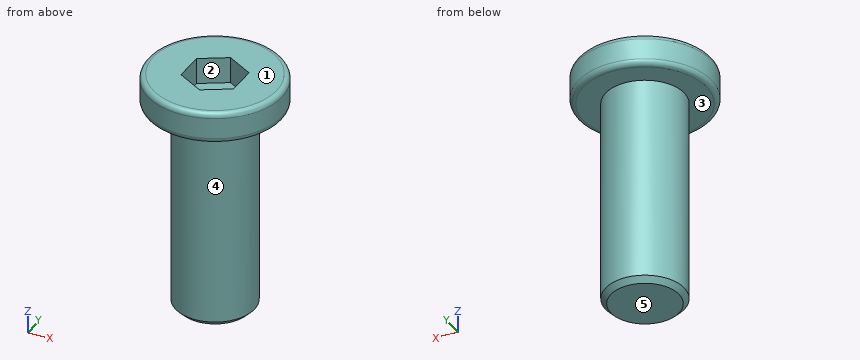
Autodesk Inventor part; units mm, degrees
ref_plane "YZ Plane" through (0, 0, 0) normal (1, 0, 0) x (0, 1, 0)
ref_plane "XZ Plane" through (0, 0, 0) normal (0, 1, 0) x (-1, 0, 0)
ref_plane "XY Plane" through (0, 0, 0) normal (0, 0, 1) x (1, 0, 0)
sketch "スケッチ1" plane through (0, 0, 0) normal (0, 0, 1) x (1, 0, 0)
  circle A0 centre (0, 0) radius 2.55
  dimension "d0" = 5.1
extrude "押し出し1" add sketch "スケッチ1" along normal blind 1.2
sketch "スケッチ2" plane through (0, 0, 0) normal (0, 0, -1) x (-1, 0, 0)
  circle A0 centre (0, 0) radius 2.55
  circle A1 centre (0, 0) radius 1.5
  dimension "d3" = 3
extrude "押し出し2" add sketch "スケッチ2" along normal blind 8 contours A1
thread "ねじ1"
sketch "スケッチ3" plane through (0, 0, 1.2) normal (0, 0, 1) x (1, 0, 0)
  circle A0 centre (0, 0) radius 2.55
  line L0 (0, 1.1547) -> (1, 0.5774)
  line L1 (1, 0.5774) -> (1, -0.5774)
  line L2 (1, -0.5774) -> (0, -1.1547)
  line L3 (0, -1.1547) -> (-1, -0.5774)
  line L4 (-1, -0.5774) -> (-1, 0.5774)
  line L5 (-1, 0.5774) -> (0, 1.1547)
  dimension "d8" = 2
extrude "押し出し3" cut sketch "スケッチ3" against normal blind 1 contours L0 L1 L2 L3 L4 L5
fillet "フィレット1" radius 0.2 2 edges at (-2.55, 0, 1.2) (-2.55, 0, 0)
chamfer "面取り1" distance 0.2 angle 45 1 edges at (1.5, 0, -8)
properties part number "六角穴付低頭平 M3 x 8" material "鋼"
Here's how the part is built. I have some questions about the finished solid (model axes, mm). Face numbers are marked on the shaded views. A direction names the side the tool comes from. Coordinates: 2 decimals unless noted, no trailing zeros. Loops run counter-clockwise (first coordinate to the right, second up) from the corner with the lowest first, then second, coordinate; pieces in that order, holes last.
1. For the marked faces 4 and 5, which set-ups out of +Z, -Z, +X, -X, +Y, -Y let a thin tool reach every point of the face, with its end or its side?
2. I need wall thicknesses on L1, parallel to X at y = -0.75, z = -5; L2, parallel to Z at x = -2.1, y = 0.2; L3, parallel to X at y = -0.9, z = 0.5. Which ranges of each line are inside material? Lowest first, please.
3. Imagine slicing it at A-A, the plane y = 0. Please give me the cut outline in (x, z), and give its area (3 significant figures).
4. If we mould it in two halves opening along Z, with no side actions, what happens to the marked faces 1, 2 and 3? For each: pulls with the +Z half, pulls with the -Z half, needs draft (parallel to the pull), parting line crosses it, or undercut.
5. Imagine slicing it at B-B, the plane z = -2.25. Please give me the cut outline in (x, y), and give its area (3 significant figures).
6. For P1, Ø3, axis at y = -1.5, z = -2.5, coming from the +X side; P2, Ø1, axis at x = 0, y = -0.5, coming from the +Z side, each with a flat end and sliding along its axis, tell me the tip position at first contact or that it passes through.
Taken from the geometry:
1. face 4: -Z
1. face 5: -Z, +X, -X, +Y, -Y
2. L1: x = -1.3 to 1.3
2. L2: z = 0 to 1.2
2. L3: x = -2.39 to -0.44, 0.44 to 2.39
3. outline: (-2.55, 0.2) arc R0.2 ccw to (-2.35, 0) - (-1.5, 0) - (-1.5, -7.8) - (-1.3, -8) - (1.3, -8) - (1.5, -7.8) - (1.5, 0) - (2.35, 0) arc R0.2 ccw to (2.55, 0.2) - (2.55, 1) arc R0.2 ccw to (2.35, 1.2) - (1, 1.2) - (1, 0.2) - (-1, 0.2) - (-1, 1.2) - (-2.35, 1.2) arc R0.2 ccw to (-2.55, 1) - close
3. area: 28.0 mm2
4. face 1: pulls with the +Z half
4. face 2: needs draft
4. face 3: pulls with the -Z half
5. outline: circle Ø3 at (0, 0)
5. area: 7.07 mm2
6. P1: stops at x = 1.5
6. P2: stops at z = 0.2
